```python
from build123d import *

# Parameters (mm, degrees)
SKETCH_1_W           = 18
SKETCH_1_H           = 9
EXTRUDE_1_DEPTH      = 8.3
SKETCH_1_12_R        = 3.5
CUT_EXTRUDE_1_DEPTH  = 6.8
SKETCH_1_14_R        = 3.5
CUT_EXTRUDE_2_DEPTH  = 5.1
SKETCH_1_15_R        = 3.5
CUT_EXTRUDE_3_DEPTH  = 3.4
SKETCH_1_16_R        = 4
CUT_EXTRUDE_4_DEPTH  = 1.7
CUT_EXTRUDE_5_DEPTH  = 5.1
CUT_EXTRUDE_6_DEPTH  = 2.9
CUT_EXTRUDE_7_DEPTH  = 1.2
SKETCH_3_W           = 5.4
SKETCH_3_H           = 6.8
CUT_EXTRUDE_8_DEPTH  = 2
SKETCH_1_19_R        = 1.5
CUT_EXTRUDE_9_DEPTH  = 6.8
CUT_EXTRUDE_10_DEPTH = 1.7
CUT_EXTRUDE_11_DEPTH = 1.2
CUT_EXTRUDE_START    = 0.5
CUT_EXTRUDE_13_DEPTH = 1.2
CUT_EXTRUDE_START_2  = 6.8
SKETCH_1_20_R        = 0.6
CUT_EXTRUDE_14_DEPTH = 15.969014677
CUT_EXTRUDE_START_3  = 1.7
SKETCH_1_21_R        = 0.75
SKETCH_1_21_R_2      = 0.6
CUT_EXTRUDE_15_DEPTH = 21.069014677
SKETCH_6_R           = 0.6
CUT_EXTRUDE_16_DEPTH = 22.179235114
SKETCH_6_3_R         = 1.5
CUT_EXTRUDE_17_DEPTH = 3.4
SKETCH_7_W           = 18
SKETCH_7_H           = 5
SKETCH_7_R           = 0.6
EXTRUDE_2_DEPTH      = 1
SKETCH_8_R           = 0.35
CUT_EXTRUDE_18_DEPTH = 2


with BuildPart() as part:
    # 草图1 → 凸台-拉伸1 (new body)
    with BuildSketch(Plane(origin=(0, 0, 0), x_dir=(0, 0, -1), z_dir=(1, 0, 0))):
        with Locations((-9, -4.5)):
            Rectangle(SKETCH_1_W, SKETCH_1_H)
    extrude(amount=EXTRUDE_1_DEPTH)

    # 草图1<12> → 切除-拉伸1 (cut)
    with BuildSketch(Plane(origin=(0, 0, 0), x_dir=(0, 0, -1), z_dir=(1, 0, 0))):
        with Locations((-14.724922359, -2.5)):
            Circle(SKETCH_1_12_R)
    extrude(amount=CUT_EXTRUDE_1_DEPTH, mode=Mode.SUBTRACT)

    # 草图1<14> → 切除-拉伸2 (cut)
    with BuildSketch(Plane(origin=(0, 0, 0), x_dir=(0, 0, -1), z_dir=(1, 0, 0))):
        with Locations((-14.724922359, -6.7)):
            Circle(SKETCH_1_14_R)
    extrude(amount=CUT_EXTRUDE_2_DEPTH, mode=Mode.SUBTRACT)

    # 草图1<15> → 切除-拉伸3 (cut)
    with BuildSketch(Plane(origin=(0, 0, 0), x_dir=(0, 0, -1), z_dir=(1, 0, 0))):
        with Locations((-10.524922359, -6.7)):
            Circle(SKETCH_1_15_R)
    extrude(amount=CUT_EXTRUDE_3_DEPTH, mode=Mode.SUBTRACT)

    # 草图1<16> → 切除-拉伸4 (cut)
    with BuildSketch(Plane(origin=(0, 0, 0), x_dir=(0, 0, -1), z_dir=(1, 0, 0))):
        with Locations((-6.5, -5.5)):
            Circle(SKETCH_1_16_R)
    extrude(amount=CUT_EXTRUDE_4_DEPTH, mode=Mode.SUBTRACT)

    # 草图1<17> → 切除-拉伸5 (cut)
    with BuildSketch(Plane(origin=(0, 0, 0), x_dir=(0, 0, -1), z_dir=(1, 0, 0))):
        with BuildLine():
            Line((-18, -9), (-17.363103551, -9))
            ThreePointArc((-17.363103551, -9), (-17.729170482, -8.495687395), (-18, -7.934449857))
            Line((-18, -7.934449857), (-18, -9))
        make_face()
        with BuildLine():
            ThreePointArc((-17.524922359, -4.6), (-17.793136229, -4.184061654), (-18, -3.734449857))
            Line((-18, -3.734449857), (-18, -5.465550143))
            ThreePointArc((-18, -5.465550143), (-17.793136229, -5.015938346), (-17.524922359, -4.6))
        make_face()
        with BuildLine():
            ThreePointArc((-18, -1.265550143), (-17.656316605, -0.58769046), (-17.174412102, 0))
            Line((-17.174412102, 0), (-18, 0))
            Line((-18, 0), (-18, -1.265550143))
        make_face()
    extrude(amount=CUT_EXTRUDE_5_DEPTH, mode=Mode.SUBTRACT)

    # 草图1<18> → 切除-拉伸6 (cut)
    with BuildSketch(Plane(origin=(0, 0, 0), x_dir=(0, 0, -1), z_dir=(1, 0, 0))):
        with BuildLine():
            Line((0, -9), (0, 0))
            Line((0, 0), (-8.624932715, 0))
            ThreePointArc((-8.624932715, 0), (-8.624924948, -0.004006417), (-8.624922359, -0.008012841))
            ThreePointArc((-8.624922359, -0.008012841), (-9.378363691, -2.033762682), (-11.272446499, -3.074813388))
            ThreePointArc((-11.272446499, -3.074813388), (-11.292201209, -3.182953516), (-11.315342274, -3.290419915))
            ThreePointArc((-11.315342274, -3.290419915), (-10.569517592, -3.200284116), (-9.821638329, -3.271386348))
            ThreePointArc((-9.821638329, -3.271386348), (-5.335215324, -1.673346546), (-2.5, -5.5))
            ThreePointArc((-2.5, -5.5), (-3.054280431, -7.531506006), (-4.563508327, -9))
            Line((-4.563508327, -9), (0, -9))
        make_face()
        with BuildLine():
            ThreePointArc((-8.624922359, -0.008012841), (-8.624924948, -0.004006417), (-8.624932715, 0))
            Line((-8.624932715, 0), (-10.224943762, 0))
            ThreePointArc((-10.224943762, 0), (-10.22492771, -0.004006406), (-10.224922359, -0.008012841))
            ThreePointArc((-10.224922359, -0.008012841), (-10.548791645, -0.938988964), (-11.380544415, -1.467945659))
            ThreePointArc((-11.380544415, -1.467945659), (-11.264046545, -1.978139294), (-11.224922359, -2.5))
            ThreePointArc((-11.224922359, -2.5), (-11.236823629, -2.788387316), (-11.272446499, -3.074813388))
            ThreePointArc((-11.272446499, -3.074813388), (-9.378363691, -2.033762682), (-8.624922359, -0.008012841))
        make_face()
        with BuildLine():
            Line((-10.224943762, 0), (-8.624932715, 0))
            ThreePointArc((-8.624932715, 0), (-11.218224886, 3.050296769), (-14.656688161, 0.999334807))
            ThreePointArc((-14.656688161, 0.999334807), (-13.853421855, 0.889762067), (-13.096913716, 0.598320167))
            ThreePointArc((-13.096913716, 0.598320167), (-11.418994363, 1.460458494), (-10.224943762, 0))
        make_face()
        with BuildLine():
            ThreePointArc((-13.096913716, 0.598320167), (-13.853421855, 0.889762067), (-14.656688161, 0.999334807))
            ThreePointArc((-14.656688161, 0.999334807), (-14.781912048, 0.50658802), (-14.824912004, 0))
            Line((-14.824912004, 0), (-13.224900957, 0))
            ThreePointArc((-13.224900957, 0), (-13.191738507, 0.305755209), (-13.096913716, 0.598320167))
        make_face()
        with BuildLine():
            ThreePointArc((-10.224922359, -0.008012841), (-10.22492771, -0.004006406), (-10.224943762, 0))
            Line((-10.224943762, 0), (-12.275432617, 0))
            ThreePointArc((-12.275432617, 0), (-11.736454222, -0.678171745), (-11.380544415, -1.467945659))
            ThreePointArc((-11.380544415, -1.467945659), (-10.548791645, -0.938988964), (-10.224922359, -0.008012841))
        make_face()
        with BuildLine():
            Line((-12.275432617, 0), (-10.224943762, 0))
            ThreePointArc((-10.224943762, 0), (-11.418994363, 1.460458494), (-13.096913716, 0.598320167))
            ThreePointArc((-13.096913716, 0.598320167), (-12.664341124, 0.329135022), (-12.275432617, 0))
        make_face()
        with BuildLine():
            ThreePointArc((-11.380544415, -1.467945659), (-11.736454222, -0.678171745), (-12.275432617, 0))
            Line((-12.275432617, 0), (-13.224900957, 0))
            ThreePointArc((-13.224900957, 0), (-12.659036556, -1.181652764), (-11.380544415, -1.467945659))
        make_face()
        with BuildLine():
            Line((-13.224900957, 0), (-12.275432617, 0))
            ThreePointArc((-12.275432617, 0), (-12.664341124, 0.329135022), (-13.096913716, 0.598320167))
            ThreePointArc((-13.096913716, 0.598320167), (-13.191738507, 0.305755209), (-13.224900957, 0))
        make_face()
    extrude(amount=CUT_EXTRUDE_6_DEPTH, mode=Mode.SUBTRACT)

    # 草图2 → 切除-拉伸7 (cut)
    with BuildSketch(Plane.ZY.offset(-1.7)):
        with BuildLine():
            ThreePointArc((6.5, -9), (3.374181267, -3.925434267), (9.31246118, -3.416718427))
            ThreePointArc((9.31246118, -3.416718427), (9.564297417, -3.334409455), (9.821638329, -3.271386348))
            ThreePointArc((9.821638329, -3.271386348), (3.553152293, -2.795173094), (4.563508327, -9))
            Line((4.563508327, -9), (6.5, -9))
        make_face()
    extrude(amount=-CUT_EXTRUDE_7_DEPTH, mode=Mode.SUBTRACT)

    # 草图3 → 切除-拉伸8 (cut)
    with BuildSketch(Plane(origin=(0, 0, 0), x_dir=(1, 0, 0), z_dir=(0, 1, 0))):
        with Locations((5.6, -3.4)):
            Rectangle(SKETCH_3_W, SKETCH_3_H)
    extrude(amount=-CUT_EXTRUDE_8_DEPTH, mode=Mode.SUBTRACT)

    # 草图1<19> → 切除-拉伸9 (cut)
    with BuildSketch(Plane(origin=(0, 0, 0), x_dir=(0, 0, -1), z_dir=(1, 0, 0))):
        with Locations((-11.724922359, -0.008012841)):
            Circle(SKETCH_1_19_R)
    extrude(amount=CUT_EXTRUDE_9_DEPTH, mode=Mode.SUBTRACT)

    # 草图4 → 切除-拉伸10 (cut)
    with BuildSketch(Plane.ZY.offset(-2.9)):
        with BuildLine():
            Line((10.224943762, 0), (6.8, 0))
            Line((6.8, 0), (6.8, -2))
            Line((6.8, -2), (6.5, -2))
            ThreePointArc((6.5, -2), (8.074565733, -2.374181267), (9.31246118, -3.416718427))
            ThreePointArc((9.31246118, -3.416718427), (10.304655394, -3.206937953), (11.315342274, -3.290419915))
            ThreePointArc((11.315342274, -3.290419915), (11.227160165, -2.374861561), (11.380544415, -1.467945659))
            ThreePointArc((11.380544415, -1.467945659), (10.546309243, -0.935844249), (10.224943762, 0))
        make_face()
    extrude(amount=-CUT_EXTRUDE_10_DEPTH, mode=Mode.SUBTRACT)

    # 草图5 → 切除-拉伸11 (cut)
    with BuildSketch(Plane.ZY.offset(-3.4)):
        with BuildLine():
            ThreePointArc((11.315342274, -3.290419915), (10.304655394, -3.206937953), (9.31246118, -3.416718427))
            ThreePointArc((9.31246118, -3.416718427), (9.45763616, -3.628533104), (9.58689031, -3.850421808))
            ThreePointArc((9.58689031, -3.850421808), (10.545192403, -3.70006848), (11.501375265, -3.863357667))
            ThreePointArc((11.501375265, -3.863357667), (11.396009855, -3.580898486), (11.315342274, -3.290419915))
        make_face()
    extrude(amount=-CUT_EXTRUDE_11_DEPTH, mode=Mode.SUBTRACT)

    # 草图5<4> → 切除-拉伸13 (cut)
    with BuildSketch(Plane.ZY.offset(-3.4).offset(CUT_EXTRUDE_START)):
        with BuildLine():
            ThreePointArc((9.31246118, -3.416718427), (3.374181267, -3.925434267), (6.5, -9))
            ThreePointArc((6.5, -9), (7.115838654, -8.945394426), (7.71246118, -8.783281573))
            ThreePointArc((7.71246118, -8.783281573), (7.567286199, -8.571466896), (7.438032049, -8.349578192))
            ThreePointArc((7.438032049, -8.349578192), (3.625055458, -4.642857143), (8.845337154, -3.629333372))
            ThreePointArc((8.845337154, -3.629333372), (9.074996723, -3.514452065), (9.31246118, -3.416718427))
        make_face()
        with BuildLine():
            ThreePointArc((7.71246118, -8.783281573), (7.115838654, -8.945394426), (6.5, -9))
            Line((6.5, -9), (7.886741168, -9))
            ThreePointArc((7.886741168, -9), (7.797447835, -8.893372453), (7.71246118, -8.783281573))
        make_face()
    extrude(amount=CUT_EXTRUDE_13_DEPTH, mode=Mode.SUBTRACT)

    # 草图1<20> → 切除-拉伸14 (cut, through all)
    with BuildSketch(Plane(origin=(0, 0, 0), x_dir=(0, 0, -1), z_dir=(1, 0, 0)).offset(CUT_EXTRUDE_START_2)):
        with Locations((-14.724922359, -2.5)):
            Circle(SKETCH_1_20_R)
    extrude(amount=CUT_EXTRUDE_14_DEPTH, mode=Mode.SUBTRACT)

    # 草图1<21> → 切除-拉伸15 (cut, through all)
    with BuildSketch(Plane(origin=(0, 0, 0), x_dir=(0, 0, -1), z_dir=(1, 0, 0)).offset(CUT_EXTRUDE_START_3)):
        with Locations(Location((-6.5, -5.5, 0), (0, 0, 177.482710398))):
            Circle(SKETCH_1_21_R)
        with Locations((-14.724922359, -6.7)):
            Circle(SKETCH_1_21_R_2)
        with Locations((-10.524922359, -6.7)):
            Circle(SKETCH_1_21_R_2)
    extrude(amount=CUT_EXTRUDE_15_DEPTH, mode=Mode.SUBTRACT)

    # 草图6 → 切除-拉伸16 (cut, through all)
    with BuildSketch(Plane(origin=(8.3, 0, 0), x_dir=(0, 0, -1), z_dir=(1, 0, 0))):
        with Locations((-1.25, -5.5)):
            Circle(SKETCH_6_R)
    extrude(amount=-CUT_EXTRUDE_16_DEPTH, mode=Mode.SUBTRACT)

    # 草图6<3> → 切除-拉伸17 (cut)
    with BuildSketch(Plane(origin=(8.3, 0, 0), x_dir=(0, 0, -1), z_dir=(1, 0, 0))):
        with Locations((-1.25, -5.5)):
            Circle(SKETCH_6_3_R)
    extrude(amount=-CUT_EXTRUDE_17_DEPTH, mode=Mode.SUBTRACT)

    # 草图7 → 凸台-拉伸2 (add)
    with BuildSketch(Plane.XY.offset(18)):
        with Locations((-0.7, -2.5)):
            Rectangle(SKETCH_7_W, SKETCH_7_H)
        with Locations((-5.7, -2.5)):
            Circle(SKETCH_7_R, mode=Mode.SUBTRACT)
        with Locations((0.6, -2.5)):
            Circle(SKETCH_7_R, mode=Mode.SUBTRACT)
    extrude(amount=EXTRUDE_2_DEPTH)

    # 草图8 → 切除-拉伸18 (cut)
    with BuildSketch(Plane(origin=(0, 0, 0), x_dir=(1, 0, 0), z_dir=(0, 1, 0))):
        with Locations(Location((6.45, -8.512471881, 0), (0, 0, 270))):
            Circle(SKETCH_8_R)
    extrude(amount=-CUT_EXTRUDE_18_DEPTH, mode=Mode.SUBTRACT)


solid = part.part
```
For this review, take the finished solid that the model builds, in its own axes (mm). A direction names the side the tool comes from. Give positions to 0.01 mm unless a question says otherwise; leave off trailing zeros. Order: outer loops, then holes, each group sorted by start corner. A loop starts at its lowest first (then second) coordinate and runs counter-clockwise, first axis right, second up.
1) For faces 5 (the face through (4.6, -2, 10)), 6 (the face through (5.94, -0.58, 17.65)), 7 (the face through (-0.8, -5, 18.5)), 8 (the face through (6, -2, 3)), 9 (the face through (1.7, -5.5, 5.6)), list the 3-axis set-ups (+Z, -Z, +X, -X, +Y, -Y) from which the entire face can be reached by the end or side of a thin tool; tool diameter is ignored.
2) Take a section at A-A (z = 1.25). Give the boundary of the cut face in (x, y), then the cut area to 3 significant figures.
3) Take a section at C-C (y = -1). Give the boundary of the cut face in (x, z), then the cut area to 3 significant figures.
4) Wall thickness on line 1 (Y direction, x = 6.9, z = 1.25); line 2 (Z direction, x = 6, y = -5.5); line 3 (Y direction, x = 4.45, z = 1.25): over which ranges is each line inside the solid? List them lowest first.
5) Take a section at B-B (x = -5.7). Give the boundary of the cut face in (y, z).
6) The part is to be moulded in two halves that separate along X. For faces 1 (the face through (3.4, -7, 9)), 2 (the face through (4.9, -5, 2)), 3 (the face through (7, -7, 18)), 4 (the face through (0.923, -1.994, 18.493)), say which applies: released by +X, released by -X, zero draft, split by the parting line, or undercut.
7) Take a section at D-D (x = 6.45). Give the boundary of the cut face in (y, z).
8) Insertion check: pin 1 (1.9 mm diameter, centred on y = -6.7, z = 10.52, fed in from +X); pin 2 (10 mm diameter, centred on x = -1.5, z = 3, fed in from +Y); pin 3 (4 mm diameter, centred on y = -2.5, z = 9.5, fed in from -X); pin 4 (4 mm diameter, centred on x = -1.5, y = -1.5, fed in from -Z). Each pin has a flat end and moves straight along its axis. Give the tip position at first contact, or say it passes through.
Derived:
1. face 5: -X, +Y
1. face 6: -X
1. face 7: +Z, +X, -X, -Y
1. face 8: -Z, +X, -X, +Y
1. face 9: -Z, -X, +Y, -Y
2. outline: (2.9, -9) - (8.3, -9) - (8.3, -7) - (4.9, -7) - (4.9, -6.1) - (2.9, -6.1) - close; (2.9, -4.9) - (4.9, -4.9) - (4.9, -4) - (8.3, -4) - (8.3, -2) - (2.9, -2) - close
2. area: 25.2 mm2
3. outline: (-9.7, 18) - (5.1, 18) - (5.1, 17.89) - (6.8, 17.89) - (6.8, 10.6) - (4.6, 10.6) - (4.6, 6.8) - (8.3, 6.8) - (8.3, 19) - (-9.7, 19) - close; hole circle Ø0.7 at (6.45, 8.51)
3. area: 43.0 mm2
4. line 1: y = -9 to -7, -4 to -2
4. line 2: z = 2.75 to 5.75, 7.25 to 12.92, 16.53 to 18
4. line 3: y = -9 to -6.1, -4.9 to -2
5. outline: (-5, 18) - (-3.1, 18) - (-3.1, 19) - (-5, 19) - close; (-1.9, 18) - (0, 18) - (0, 19) - (-1.9, 19) - close
6. face 1: released by -X
6. face 2: released by +X
6. face 3: zero draft
6. face 4: undercut
7. outline: (-9, 0) - (-6.33, 0) arc R1.5 cw (long way) to (-4.67, 0) - (-2, 0) - (-2, 6.8) - (0, 6.8) - (0, 8.16) - (-2, 8.16) - (-2, 8.86) - (0, 8.86) - (0, 10.22) arc R1.5 cw to (-1.47, 11.38) arc R3.5 cw to (-3.73, 18) - (-1.27, 18) arc R3.5 cw to (0, 17.17) - (0, 19) - (-5, 19) - (-5, 18) - (-9, 18) - close; hole circle Ø1.2 at (-6.7, 10.52); hole circle Ø1.2 at (-6.7, 14.72); hole circle Ø1.5 at (-5.5, 6.5)
8. pin 1: stops at x = 8.3
8. pin 2: stops at y = -2
8. pin 3: stops at x = 1.7
8. pin 4: stops at z = 18
